The listing builds one solid part. Answer for the finished solid, in the listing's coordinates (mm). A direction names the side the tool comes from. Round coordinates to 2 decimals unless told otherwise and drop trailing zeros. Write each loop counter-clockwise with the first axis right and the second up, starting at its lowest first coordinate (ties: lowest second). Pieces come first, ordered by that corner, then holes. Notation, with made-up numbers: M 82.5,56.5 L 109.5,56.5 A22 cw 109.5,76.5 Z; hole C 32,72 d4. An arc over 180 degrees is marked long. Write each question's results on one line, items separated by ' | '.
from build123d import *

# Parameters (mm, degrees)
F1_DEPTH      = 38.1
F3_DEPTH      = 38.1
F5_DEPTH      = 0.6731
F5_DEPTH_BACK = 0.6858


with BuildPart() as f1:
    # F0 (on Front) → F1 (new body)
    with BuildSketch(Plane.XZ):
        with BuildLine():
            Line((-17.6997391722, 33.1053871185), (-20.9649930975, 16.5606186919))
            ThreePointArc((-20.9649930975, 16.5606186919), (-14.7446558469, -2.1547528437), (0, -15.2525714094))
            ThreePointArc((0, -15.2525714094), (14.7446558469, -2.1547528437), (20.9649930975, 16.5606186919))
            Line((20.9649930975, 16.5606186919), (17.6997391722, 33.1053871185))
            Line((17.6997391722, 33.1053871185), (13.5980615388, 26.6233030993))
            Line((13.5980615388, 26.6233030993), (0, 21.6528698802))
            Line((0, 21.6528698802), (-13.5980615388, 26.6233030993))
            Line((-13.5980615388, 26.6233030993), (-17.6997391722, 33.1053871185))
        make_face()
    extrude(amount=F1_DEPTH)

    # F2 (on face) → F3 (cut)
    with BuildSketch(Plane.XZ.offset(38.1)):
        with BuildLine():
            Line((7.7268123423, 17.8562299685), (2.667, 14.0194606165))
            ThreePointArc((2.667, 14.0194606165), (6.9408367243, 13.6380038042), (7.7268123423, 17.8562299685))
        make_face()
        with BuildLine():
            Line((-2.667, 14.0194606165), (-7.7777689272, 17.7880864898))
            ThreePointArc((-7.7777689272, 17.7880864898), (-6.8829468537, 13.6518252435), (-2.667, 14.0194606165))
        make_face()
    extrude(amount=-F3_DEPTH, mode=Mode.SUBTRACT)

    # F4 (on face) → F5 (join, two sides)
    with BuildSketch(Plane.XZ.offset(38.1)) as f5_sk:
        with BuildLine():
            Line((2.220712835, 22.3098099232), (3.7018435542, 22.8101927787))
            ThreePointArc((3.7018435542, 22.8101927787), (3.6855396388, 22.9019358085), (3.6670169682, 22.9932567362))
            Line((3.6670169682, 22.9932567362), (2.2124818439, 22.461587595))
            ThreePointArc((2.2124818439, 22.461587595), (2.2179440641, 22.3857717928), (2.220712835, 22.3098099232))
        make_face()
        with BuildLine():
            Line((2.2124818439, 22.461587595), (3.6670169682, 22.9932567362))
            ThreePointArc((3.6670169682, 22.9932567362), (-0.0595272983, 26.0276638545), (-3.8353356865, 23.0547814577))
            Line((-3.8353356865, 23.0547814577), (-2.0586373149, 22.4053535535))
            ThreePointArc((-2.0586373149, 22.4053535535), (0.0508779389, 24.4116036609), (2.2124818439, 22.461587595))
        make_face()
        with BuildLine():
            Line((-2.0586373149, 22.4053535535), (-3.8353356865, 23.0547814577))
            ThreePointArc((-3.8353356865, 23.0547814577), (-3.8616258801, 22.9328813979), (-3.8839485496, 22.8101927787))
            Line((-3.8839485496, 22.8101927787), (-2.0625579637, 22.2297497094))
            ThreePointArc((-2.0625579637, 22.2297497094), (-2.0623983648, 22.3175918356), (-2.0586373149, 22.4053535535))
        make_face()
    extrude(amount=F5_DEPTH)
    extrude(f5_sk.sketch, amount=-F5_DEPTH_BACK)


solid = f1.part
1) A tool of negligible diameter and unlimited length cuts with its end or side. For faces 1 (the face through (0, -37.414, 25)), 2 (the face through (5.232, -19.317, 15.965)), 3 (the face through (19.355, -18.783, 24.717)), 4 (the face through (15.68, -18.78, 29.91)), from which of +Z, -Z, +X, -X, +Y, -Y can it reach the whole face along a straight path? Write none if from no direction.
Return value:
face 1: +Z, +Y | face 2: +Y, -Y | face 3: +Z, +X, +Y, -Y | face 4: +Z, +Y, -Y
2) Section C-C (x = 6.5) is taken. Determine the outline of the cut face in (y, z), then the cut area to 3 significant figures.
Return value:
outline: M -38.1,-11.13 L 0,-11.13 L 0,13.36 L -38.1,13.36 Z; M -38.1,16.93 L 0,16.93 L 0,24.03 L -38.1,24.03 Z | area: 1,200 mm²
3) Each of these flat-tipped pins is pushed along its axis until it touches: pin 1 (6 mm diameter, centred on x = 13.5, y = -28, fed in from -Z); pin 2 (1 mm diameter, centred on y = -12.5, z = 18.5, fed in from +X); pin 3 (3 mm diameter, centred on y = -9.5, z = 13, fed in from +X). Where does it stop, or does it pass through?
Return value:
pin 1: z = -7.49 | pin 2: x = 20.68 | pin 3: x = 20.79
4) Find the intervals of material crossed by line 1 (X direction, y = -2.5, z = 14.5); line 2 (Z direction, x = 0, y = -23); line 3 (Y direction, x = 12, z = 11), in increasing order.
Return value:
line 1: -20.79 to -7.68, -3.32 to 3.3, 7.73 to 20.79 | line 2: -15.25 to 21.65 | line 3: -38.1 to 0
5) Section D-D (z = -5) is taken. Determine the outline of the cut face in (x, y), then the cut area to 3 significant figures.
Return value:
outline: M -12.68,-38.1 L 12.68,-38.1 L 12.68,0 L -12.68,0 Z | area: 966 mm²
6) Section B-B (z = 29.5) is taken. Determine the outline of the cut face in (x, y), then the cut area to 3 significant figures.
Return value:
outline: M -18.41,-38.1 L -15.42,-38.1 L -15.42,0 L -18.41,0 Z; M 15.42,-38.1 L 18.41,-38.1 L 18.41,0 L 15.42,0 Z | area: 228 mm²
7) The mould has two halves that part along Z. Classify faces 5 (the face through (-15.62, -18.78, 29.82)), 6 (the face through (-14.9, -18.78, -1.92)), 7 (the face through (6.89, -19.32, 13.6)), 8 (the face through (0, 0, 9)): +Z half, -Z half, draft (parallel to the pull), parting line (faces both ways), or undercut.
Return value:
face 5: +Z half | face 6: -Z half | face 7: undercut | face 8: draft
8) Section A-A (y = -7.5) is taken. Determine the outline of the cut face in (x, z) (3 decimals), then the cut area to 3 significant figures.
Return value:
outline: M -20.965,16.561 A38.1 ccw 0,-15.253 A38.1 ccw 20.965,16.561 L 17.7,33.105 L 13.598,26.623 L 0,21.653 L -13.598,26.623 L -17.7,33.105 Z; hole M -7.778,17.788 A3.2 ccw -2.667,14.019 Z; hole M 2.667,14.019 A3.189 ccw 7.727,17.856 Z | area: 1,270 mm²
